```python
from build123d import *

# Parameters (mm, degrees)
SKETCH_1_W                        = 20
SKETCH_1_H                        = 60
EXTRUDE_1_DEPTH                   = 6
SKETCH_2_W                        = 7
SKETCH_2_H                        = 7
CUT_EXTRUDE_1_DEPTH               = 10
HOLE_WIZARD_4_1_4_1_1_D           = 4.1
HOLE_WIZARD_4_1_4_1_1_CSINK_D     = 4.15
HOLE_WIZARD_4_1_4_1_1_CSINK_ANGLE = 90


with BuildPart() as part:
    # 草图1 → 凸台-拉伸1 (new body)
    with BuildSketch(Plane.XY):
        Rectangle(SKETCH_1_W, SKETCH_1_H)
    extrude(amount=EXTRUDE_1_DEPTH)

    # 草图2 → 切除-拉伸1 (cut)
    with BuildSketch(Plane.XY.offset(6)):
        with Locations((0, 20)):
            Rectangle(SKETCH_2_W, SKETCH_2_H)
    cut_extrude_1 = extrude(amount=-CUT_EXTRUDE_1_DEPTH, mode=Mode.SUBTRACT)

    # 镜向1: 切除-拉伸1 across plane
    add(cut_extrude_1.mirror(Plane.ZX), mode=Mode.SUBTRACT)

    # Ø4.1 (4.1) 直径孔1 (through all)
    with Locations(Plane(origin=(-7.5, 7.5, 6), x_dir=(1, 0, 0), z_dir=(0, 0, 1))):
        with Locations((0, 0), (15, 0), (15, -15), (0, -15)):
            CounterSinkHole(HOLE_WIZARD_4_1_4_1_1_D / 2, HOLE_WIZARD_4_1_4_1_1_CSINK_D / 2, counter_sink_angle=HOLE_WIZARD_4_1_4_1_1_CSINK_ANGLE)


solid = part.part
```
Part model, mm, in its own coordinate system. A direction names the side the tool comes from. Round coordinates to 2 decimals unless told otherwise and drop trailing zeros. Write each loop counter-clockwise with the first axis right and the second up, starting at its lowest first coordinate (ties: lowest second). Pieces come first, ordered by that corner, then holes. Notation, with made-up numbers: (28, 64) -> (50, 64) arc R16 cw to (50, 72) -> close; hole circle Ø7 at (-29.75, 23.5). An arc over 180 degrees is marked (long way). Return JSON: item names as keys, results as strings. Group by question number.
Q1. Probe L1, parallel to Y at x = 1, z = 0.95; L2, parallel to Y at x = -7.5, z = 3.9; L3, parallel to X at y = -7.5, z = 1.95. List the from-to ranges inside material, lowest first. Write a range as [from, to].
Q2. Saw through at B-B on x = -7.5. Write the cut outline in (y, z) (3 decimals), plus the area to 3 significant figures.
Q3. Saw through at C-C on z = 4.2. Write the cut outline in (x, y).
Q4. Mould opens along Y. For faces 1 (the flat face through (-3.5, -20, 3)), 2 (the flat face through (0, 0, 6)), 3 (the cylindrical face through (-5.45, -7.41, 2.95)), 4 (the flat face through (0, -30, 3)) say: pulls with the +Y half, pulls with the -Y half, needs draft (parallel to the pull), parting line crosses it, or undercut.
Q5. Saw through at A-A on y = 7.5. Write the cut outline in (x, z) (3 decimals).
Q6. Pin check, flat tip, straight feed: pin 1 (6.5 mm diameter, centred on x = -7.5, y = 7.5, fed in from +Z). Stop position of the tip, or through.
Q7. Which spindle directions (+Z, -Z, +X, -X, +Y, -Y) get a long thin tool onto all of the face, cutting with end or side? Do faces 5 (the flat face through (-3.5, 20, 3)), 6 (the flat face through (10, 0, 3)). Say none if no direction does.
Q8. Saw through at D-D on y = 22. Write the cut outline in (x, z), plus the area to 3 significant figures.
Answer:
{
 "1": {"L1": "[-30, -23.5], [-16.5, 16.5], [23.5, 30]", "L2": "[-30, -9.55], [-5.45, 5.45], [9.55, 30]", "L3": "[-10, -9.55], [-5.45, 5.45], [9.55, 10]"},
 "2": {"outline": "(-30, 0) -> (-9.55, 0) -> (-9.55, 5.975) -> (-9.575, 6) -> (-30, 6) -> close; (-5.45, 0) -> (5.45, 0) -> (5.45, 5.975) -> (5.425, 6) -> (-5.425, 6) -> (-5.45, 5.975) -> close; (9.55, 0) -> (30, 0) -> (30, 6) -> (9.575, 6) -> (9.55, 5.975) -> close", "area": "311 mm2"},
 "3": {"outline": "(-10, -30) -> (10, -30) -> (10, 30) -> (-10, 30) -> close; hole circle Ø4.1 at (-7.5, -7.5); hole circle Ø4.1 at (-7.5, 7.5); hole (-3.5, -23.5) -> (3.5, -23.5) -> (3.5, -16.5) -> (-3.5, -16.5) -> close; hole (-3.5, 16.5) -> (3.5, 16.5) -> (3.5, 23.5) -> (-3.5, 23.5) -> close; hole circle Ø4.1 at (7.5, -7.5); hole circle Ø4.1 at (7.5, 7.5)"},
 "4": {"face 1": "undercut", "face 2": "needs draft", "face 3": "undercut", "face 4": "pulls with the -Y half"},
 "5": {"outline": "(-10, 0) -> (-9.55, 0) -> (-9.55, 5.975) -> (-9.575, 6) -> (-10, 6) -> close; (-5.45, 0) -> (5.45, 0) -> (5.45, 5.975) -> (5.425, 6) -> (-5.425, 6) -> (-5.45, 5.975) -> close; (9.55, 0) -> (10, 0) -> (10, 6) -> (9.575, 6) -> (9.55, 5.975) -> close"},
 "6": {"pin 1": "z = 6"},
 "7": {"face 5": "+Z, -Z", "face 6": "+Z, -Z, +X, +Y, -Y"},
 "8": {"outline": "(-10, 0) -> (-3.5, 0) -> (-3.5, 6) -> (-10, 6) -> close; (3.5, 0) -> (10, 0) -> (10, 6) -> (3.5, 6) -> close", "area": "78.0 mm2"}
}
